from build123d import *

# Parameters (mm, degrees)
F1_DEPTH = 31.242
F2_R     = 12.75
F3_DEPTH = 6.35
F5_DEPTH = 25.4
F7_DEPTH = 3.048


with BuildPart() as f1:
    # F0 (on Top) → F1 (new body)
    with BuildSketch(Plane.XY):
        with BuildLine():
            Line((-43.664057, -7.965392), (16.06224, -7.965392))
            Line((16.06224, -7.965392), (26.521553, -7.965392))
            Line((26.521553, -7.965392), (10.554898, 0))
            Line((10.554898, 0), (-42.705316, 0))
            ThreePointArc((-42.705316, 0), (-53.620007, 23.957304), (-42.705316, 47.914608))
            Line((-42.705316, 47.914608), (16.06224, 47.914608))
            Line((16.06224, 47.914608), (16.06224, 55.534608))
            Line((16.06224, 55.534608), (-43.664057, 55.534608))
            ThreePointArc((-43.664057, 55.534608), (-62.468951, 23.784608), (-43.664057, -7.965392))
        make_face()
    extrude(amount=F1_DEPTH)

    # F2 (on face) → F3 (cut)
    with BuildSketch(Plane(origin=(0, 55.534608, 0), x_dir=(-1, 0, 0), z_dir=(0, 1, 0))):
        with Locations((0, 14.851301)):
            Circle(F2_R)
    extrude(amount=-F3_DEPTH, mode=Mode.SUBTRACT)

    # F4 (on face) → F5 (cut)
    with BuildSketch(Plane(origin=(0, 49.184608, 0), x_dir=(-1, 0, 0), z_dir=(0, 1, 0))):
        with BuildLine():
            ThreePointArc((12.75, 14.851301), (12.626213, 16.623652), (12.257258, 18.361589))
            Line((12.257258, 18.361589), (7.501453, 18.361589))
            Line((7.501453, 18.361589), (7.501453, 12.011589))
            Line((7.501453, 12.011589), (12.429744, 12.011589))
            ThreePointArc((12.429744, 12.011589), (12.669683, 13.422444), (12.75, 14.851301))
        make_face()
    extrude(amount=-F5_DEPTH, mode=Mode.SUBTRACT)

    # F6 (on face) → F7 (cut)
    with BuildSketch(Plane.XZ.offset(-47.914608)):
        Polygon((-12.429744, 12.011589), (-12.257258, 18.361589), (-42.705316, 18.361589), (-42.705316, 12.011589), align=None)
    extrude(amount=-F7_DEPTH, mode=Mode.SUBTRACT)


solid = f1.part
CAD build for the part. Positions are in the model's coordinates, mm. A direction names the side the tool comes from. Give positions to 0.01 mm unless a question says otherwise; leave off trailing zeros. Write each loop counter-clockwise with the first axis right and the second up, starting at its lowest first coordinate (ties: lowest second). Pieces come first, ordered by that corner, then holes. Notation, with made-up numbers: (35.25, 29) -> (71.25, 29) arc R25 cw to (71.25, 57) -> close; hole circle Ø5 at (8.25, 73). An arc over 180 degrees is marked (long way). Return JSON: item names as keys, results as strings.
Item 1: Band-saw the part on A-A (x = 0). List the corners of the cut face in (y, z).
Answer below:
{"outline": "(-7.97, 0) -> (0, 0) -> (0, 31.24) -> (-7.97, 31.24) -> close; (47.91, 0) -> (55.53, 0) -> (55.53, 2.1) -> (49.18, 2.1) -> (49.18, 27.6) -> (55.53, 27.6) -> (55.53, 31.24) -> (47.91, 31.24) -> close"}
Item 2: Tool access for faces 5 (the flat face through (16.062, 52, 15)), 6 (the flat face through (0, 49.185, 15)), 7 (the flat face through (18.65, -4.04, 15.4)), 8 (the flat face through (-25, 49, 12.012)), 9 (the flat face through (-20, 55.535, 15)): list every direction of +Z, -Z, +X, -X, +Y, -Y with a clear straight run to the whole face (end or side of a thin tool).
Answer below:
{"face 5": "+Z, -Z, +X, +Y", "face 6": "+Y", "face 7": "+Z, -Z, +X", "face 8": "none", "face 9": "+Z, -Z, +X, -X, +Y"}
Item 3: Band-saw the part on B-B (z = 7). List the corners of the cut face in (x, y), then the cut area to 3 significant figures.
Answer below:
{"outline": "(-43.66, -7.97) -> (26.52, -7.97) -> (10.55, 0) -> (-42.71, 0) arc R31.75 cw to (-42.71, 47.91) -> (16.06, 47.91) -> (16.06, 55.53) -> (10.05, 55.53) -> (10.05, 49.18) -> (-10.05, 49.18) -> (-10.05, 55.53) -> (-43.66, 55.53) arc R36.21 ccw to start", "area": "1,360 mm2"}
Item 4: Band-saw the part on D-D (z = 11). List the corners of the cut face in (x, y).
Answer below:
{"outline": "(-43.66, -7.97) -> (26.52, -7.97) -> (10.55, 0) -> (-42.71, 0) arc R31.75 cw to (-42.71, 47.91) -> (16.06, 47.91) -> (16.06, 55.53) -> (12.15, 55.53) -> (12.15, 49.18) -> (-12.15, 49.18) -> (-12.15, 55.53) -> (-43.66, 55.53) arc R36.21 ccw to start"}
Item 5: Drop flat-ended pins along their axis: pin 1 (3.5 mm diameter, centred on y = 50, z = 14.5, fed in from +X); pin 2 (6 mm diameter, centred on y = 31.5, z = 21.5, fed in from +X); pin 3 (5 mm diameter, centred on y = 46.5, z = 26, fed in from -X). Give the stop position or say it passes through.
Answer below:
{"pin 1": "stops at x = 16.06", "pin 2": "stops at x = -51.82", "pin 3": "stops at x = -56.3"}
Item 6: Drill centre lines: probe 1 along Y at (x, z) = (3, 14); probe 2 along Y at (x, z) = (-32, 27.5); probe 3 along Z at (x, y) = (0, 52). Where is each one in solid material? Low to high.
Answer below:
{"probe 1": "y = -7.97 to 0, 47.91 to 49.18", "probe 2": "y = -7.97 to 0, 47.91 to 55.53", "probe 3": "z = 0 to 2.1, 27.6 to 31.24"}
Item 7: Band-saw the part on C-C (y = 44). List the corners of the cut face in (x, z), then the cut area to 3 significant figures.
Answer below:
{"outline": "(-56.3, 0) -> (-46.49, 0) -> (-46.49, 31.24) -> (-56.3, 31.24) -> close", "area": "306 mm2"}
Item 8: Two-plate mould, pull along X, no slides. Class faces 1 (the flat face through (-28, 50.963, 15)), 2 (the flat face through (-16, 0, 15)), 3 (the cylindrical face through (2.764, 52.404, 2.404)), 4 (the cylindrical face through (-53.618, 23.577, 15.402)): +X half, -X half, draft (parallel to the pull), parting line (faces both ways), or undercut.
Answer below:
{"face 1": "undercut", "face 2": "draft", "face 3": "undercut", "face 4": "+X half"}
